from build123d import *

# Parameters (mm, degrees)
F0_W      = 116
F0_H      = 39
F1_DEPTH  = 30
F3_DEPTH  = 121.2
F4_W      = 116
F4_H      = 41.7851648316
F5_DEPTH  = 10
F6_W      = 101
F6_H      = 31.0710200029
F7_DEPTH  = 3
F8_R      = 1.7573065985
F9_DEPTH  = 25
F10_W     = 2
F10_H     = 1
F11_DEPTH = 3


with BuildPart() as f1:
    # F0 (on Top) → F1 (new body)
    with BuildSketch(Plane.XY):
        with Locations((-10.4412920773, -4.4543696198)):
            Rectangle(F0_W, F0_H)
        Polygon((-59.9383048147, -18.9543696198), (-59.9383048147, 10.0456303802), (-46.5383048147, 10.0456303802), (-46.5383048147, -4.4543696198), (-46.5383048147, -18.9543696198), align=None, mode=Mode.SUBTRACT)
        Polygon((-38.0383048147, -18.9543696198), (-38.0383048147, -4.4543696198), (-38.0383048147, 10.0456303802), (-24.6383048147, 10.0456303802), (-24.6383048147, -4.4543696198), (-24.6383048147, -18.9543696198), align=None, mode=Mode.SUBTRACT)
        Polygon((-16.1383048147, -18.9543696198), (-16.1383048147, -4.4543696198), (-16.1383048147, 10.0456303802), (-2.7383048147, 10.0456303802), (-2.7383048147, -4.4543696198), (-2.7383048147, -18.9543696198), align=None, mode=Mode.SUBTRACT)
        Polygon((5.7616951853, -18.9543696198), (5.7616951853, -4.4543696198), (5.7616951853, 10.0456303802), (19.1616951853, 10.0456303802), (19.1616951853, -4.4543696198), (19.1616951853, -18.9543696198), align=None, mode=Mode.SUBTRACT)
        Polygon((27.6616951853, -18.9543696198), (27.6616951853, -4.4543696198), (27.6616951853, 10.0456303802), (41.0616951853, 10.0456303802), (41.0616951853, -18.9543696198), align=None, mode=Mode.SUBTRACT)
    extrude(amount=F1_DEPTH)

    # F2 (on face) → F3 (cut)
    with BuildSketch(Plane(origin=(-68.4412920773, 0, 0), x_dir=(0, -1, 0), z_dir=(-1, 0, 0))):
        Polygon((23.9543696198, 15), (-15.0456303802, 0), (23.9543696198, 0), align=None)
    extrude(amount=-F3_DEPTH, mode=Mode.SUBTRACT)

    # F4 (on face) → F5 (join)
    with BuildSketch(Plane(origin=(0, 1.9388698944, 5.0410617253), x_dir=(1, 0, 0), z_dir=(0, -0.3589790793, -0.9333456062))):
        with Locations((-10.4412920773, 6.8498094078)):
            Rectangle(F4_W, F4_H)
        Polygon((41.0616951853, 22.3853194093), (41.0616951853, -8.6857005937), (27.6616951853, -8.6857005937), (19.1616951853, -8.6857005937), (5.7616951853, -8.6857005937), (-2.7383048147, -8.6857005937), (-16.1383048147, -8.6857005937), (-24.6383048147, -8.6857005937), (-38.0383048147, -8.6857005937), (-46.5383048147, -8.6857005937), (-59.9383048147, -8.6857005937), (-59.9383048147, 22.3853194093), (-46.5383048147, 22.3853194093), (-38.0383048147, 22.3853194093), (-24.6383048147, 22.3853194093), (-16.1383048147, 22.3853194093), (-2.7383048147, 22.3853194093), (5.7616951853, 22.3853194093), (19.1616951853, 22.3853194093), (27.6616951853, 22.3853194093), align=None, mode=Mode.SUBTRACT)
    extrude(amount=F5_DEPTH)

    # F6 (on face) → F7 (join)
    with BuildSketch(Plane(origin=(0, -1.6509208987, -4.2923943367), x_dir=(1, 0, 0), z_dir=(0, -0.3589790793, -0.9333456062))):
        with Locations((-9.4383048147, 6.8498094078)):
            Rectangle(F6_W, F6_H)
    extrude(amount=-F7_DEPTH)

    # F8 (on face) → F9 (cut)
    with BuildSketch(Plane(origin=(-68.4412920773, 0, 0), x_dir=(0, -1, 0), z_dir=(-1, 0, 0))):
        with Locations((-5.6000736372, -0.6527514918)):
            Circle(F8_R)
        with Locations((0, 1.501122984)):
            Circle(F8_R)
        with Locations((5.890285937, 3.7666175752)):
            Circle(F8_R)
        with Locations((11.5189812237, 5.9315003778)):
            Circle(F8_R)
        with Locations((17.8498418632, 8.3664467776)):
            Circle(F8_R)
    extrude(amount=-F9_DEPTH, mode=Mode.SUBTRACT)

    # F10 (on face) → F11 (join)
    with BuildSketch(Plane.XY.offset(30)):
        Polygon((35.3373080328, 9.0456303802), (33.3373080328, 9.0456303802), (28.6616951853, 9.0456303802), (28.6616951853, -17.9543696198), (33.3373080328, -17.9543696198), (35.3373080328, -17.9543696198), (40.0616951853, -17.9543696198), (40.0616951853, 9.0456303802), align=None)
        Polygon((13.4860823378, 9.0456303802), (11.4860823378, 9.0456303802), (6.7616951853, 9.0456303802), (6.7616951853, -17.9543696198), (11.4860823378, -17.9543696198), (13.4860823378, -17.9543696198), (18.1616951853, -17.9543696198), (18.1616951853, 9.0456303802), align=None)
        with Locations((12.4860823378, 9.5456303802)):
            Rectangle(F10_W, F10_H)
        with Locations((34.3373080328, 9.5456303802)):
            Rectangle(F10_W, F10_H)
        with Locations((12.4860823378, -18.4543696198)):
            Rectangle(F10_W, F10_H)
        with Locations((34.3373080328, -18.4543696198)):
            Rectangle(F10_W, F10_H)
    extrude(amount=-F11_DEPTH)


solid = f1.part
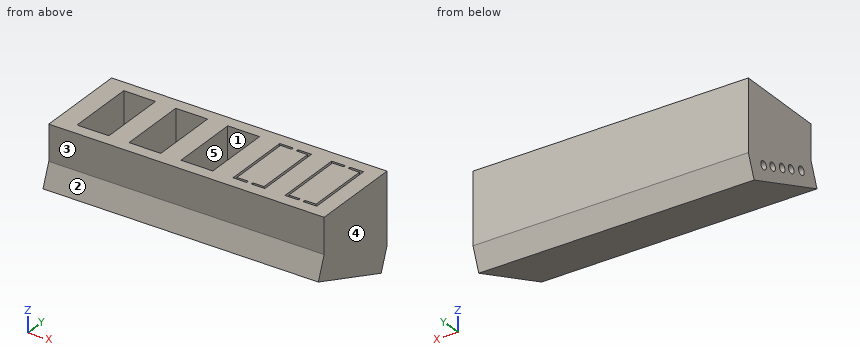
Check sheet for the modelled part. Datum: model origin and axes. Units: mm. Face numbers are marked on the shaded views. A direction names the side the tool comes from. Round coordinates to 2 decimals unless told otherwise and drop trailing zeros. Order: outer loops, then holes, each group sorted by start corner. A loop starts at its lowest first (then second) coordinate and runs counter-clockwise, first axis right, second up. Notation, with made-up numbers: M 55.5,69 L 92.5,69 A33 cw 92.5,99 Z; hole C -9.5,7.25 d8. An arc over 180 degrees is marked long. One line per item, written item: value. Start each with the question number.
1. Scan lines: line 1 along X through (y, z) = (9, 19); line 2 along X through (y, z) = (-13.5, 7.5); line 3 along Y through (x, z) = (40, 22.5). Record each from-to range of solid material in increasing order.
2. Section check A-A on x = -52. Enter the section's corners in (y, z).
3. Access from +Z, -Z, +X, -X, +Y, -Y to the whole of each face (thin tool, end or side, straight path). Record for the marked faces 1 and 2.
4. Section check B-B on z = 24. Enter the section's corners in (x, y).
5. Gauge pin test, flat ends, axial feed: P1, Ø1, axis at x = 7, y = -7, coming from the -Z side; P2, Ø1, axis at x = -49.5, z = 21, coming from the -Y side; P3, Ø10.5, axis at x = -55.5, z = 19.5, coming from the -Y side; P4, Ø4, axis at y = -19, z = 8, coming from the -X side. Record the tip position at first contact, or that the pin passes through.
6. Release check for a two-part mould opening along Y. For the marked faces 3, 4 and 5 record: released by +Y, released by -Y, zero draft, split by the parting line, or undercut.
7. Section check C-C on y = 0. Give the number of separate pieces and of enclosed holes in the cut face, and give its area (3 significant figures).
Results found:
1. line 1: -68.44 to -59.94, -46.54 to -38.04, -24.64 to -16.14, -2.74 to 5.76, 19.16 to 27.66, 41.06 to 47.56
1. line 2: -68.44 to -59.94, 41.06 to 47.56
1. line 3: -23.95 to -18.95, 10.05 to 15.05
2. outline: M -27.54,5.67 L 11.46,-9.33 L 15.05,0 L 15.05,30 L 10.05,30 L 10.05,1.92 L 7.53,-4.61 L -21.47,6.54 L -18.95,13.08 L -18.95,30 L -23.95,30 L -23.95,15 Z
3. face 1: +Z
3. face 2: +Z, +X, -X, -Y
4. outline: M -68.44,-23.95 L 47.56,-23.95 L 47.56,15.05 L -68.44,15.05 Z; hole M -59.94,-18.95 L -46.54,-18.95 L -46.54,10.05 L -59.94,10.05 Z; hole M -38.04,-18.95 L -24.64,-18.95 L -24.64,10.05 L -38.04,10.05 Z; hole M -16.14,-18.95 L -2.74,-18.95 L -2.74,10.05 L -16.14,10.05 Z; hole M 5.76,-18.95 L 19.16,-18.95 L 19.16,10.05 L 5.76,10.05 Z; hole M 27.66,-18.95 L 41.06,-18.95 L 41.06,10.05 L 27.66,10.05 Z
5. P1: z = -2.43
5. P2: y = -23.95
5. P3: y = -24.24
5. P4: x = -68.44
6. face 3: released by -Y
6. face 4: zero draft
6. face 5: undercut
7. separate pieces: 8
7. enclosed holes: 0
7. area: 1,710 mm^2
